from build123d import *

# Parameters (mm, degrees)
SKETCH1_R               = 387.5
BOSS_EXTRUDE1_DEPTH     = 62
SKETCH3_R               = 17.4625
CUT_EXTRUDE1_DEPTH      = 552.503853114
SKETCH2_R               = 292.1
BOSS_EXTRUDE2_DEPTH     = 1.5
CIRPATTERN1_COUNT       = 24
CUT_EXTRUDE4_DEPTH      = 552.67449642
CUT_EXTRUDE4_DEPTH_BACK = 552.67449642
SKETCH8_R               = 292.1


with BuildPart() as part:
    # Sketch1 → Boss-Extrude1 (new body)
    with BuildSketch(Plane.XY):
        Circle(SKETCH1_R)
    extrude(amount=BOSS_EXTRUDE1_DEPTH)

    # Sketch3 → Cut-Extrude1 (cut, symmetric)
    with BuildSketch(Plane.XY.offset(62)):
        with Locations((0, 342.9)):
            Circle(SKETCH3_R)
    cut_extrude1 = extrude(amount=CUT_EXTRUDE1_DEPTH, both=True, mode=Mode.SUBTRACT)

    # Sketch2 → Boss-Extrude2 (add)
    with BuildSketch(Plane.XY.offset(62)):
        Circle(SKETCH2_R)
    extrude(amount=BOSS_EXTRUDE2_DEPTH)

    # CirPattern1: Cut-Extrude1 ×24 about axis
    cirpattern1_axis = Axis((0, 0, 0), (0, 0, 1))
    for i in range(1, CIRPATTERN1_COUNT):
        add(cut_extrude1.rotate(cirpattern1_axis, i * 360 / CIRPATTERN1_COUNT), mode=Mode.SUBTRACT)

    # Sketch8 → Cut-Extrude4 (cut, two sides: drawn at the far end of the back side and taken through both)
    with BuildSketch(Plane.XY.offset(63.5).offset(-CUT_EXTRUDE4_DEPTH_BACK)):
        Circle(SKETCH8_R)
    extrude(amount=CUT_EXTRUDE4_DEPTH + CUT_EXTRUDE4_DEPTH_BACK, mode=Mode.SUBTRACT)


solid = part.part
CAD build for the part. Positions are in the model's coordinates, mm. Coordinates: 2 decimals unless noted, no trailing zeros. Order: outer loops, then holes, each group sorted by start corner. A loop starts at its lowest first (then second) coordinate and runs counter-clockwise, first axis right, second up.
Item 1: Pin check, flat tips, straight feed: pin 1 Ø21 at (x, y) = (331.22, 88.75) entering from +Z; pin 2 Ø3 at (x, z) = (82.5, 55.5) entering from -Y; pin 3 Ø5 at (y, z) = (301, 14) entering from +X; pin 4 Ø1 at (x, z) = (247, 27) entering from +Y. Stop position of each tip, or through.
Check sheet entries:
pin 1: passes through
pin 2: stops at y = -378.94
pin 3: stops at x = 247.09
pin 4: stops at y = 298.99
Item 2: Band-saw the part on C-C on z = 41. Give the number of separate pieces and of enclosed holes in the cut face, plus the area to 3 significant figures.
Check sheet entries:
separate pieces: 1
enclosed holes: 25
area: 181,000 mm2
Item 3: Band-saw the part on A-A on x = 0. List the corners of the cut face in (y, z), plus the area to 3 significant figures.
Check sheet entries:
outline: (-387.5, 0) - (-360.36, 0) - (-360.36, 62) - (-387.5, 62) - close; (-325.44, 0) - (-292.1, 0) - (-292.1, 62) - (-325.44, 62) - close; (292.1, 0) - (325.44, 0) - (325.44, 62) - (292.1, 62) - close; (360.36, 0) - (387.5, 0) - (387.5, 62) - (360.36, 62) - close
area: 7,500 mm2
Item 4: Band-saw the part on B-B on y = -171.45. List the corners of the cut face in (x, z), plus the area to 3 significant figures.
Check sheet entries:
outline: (-347.51, 0) - (-314.42, 0) - (-314.42, 62) - (-347.51, 62) - close; (-279.5, 0) - (-236.49, 0) - (-236.49, 62) - (-279.5, 62) - close; (236.49, 0) - (279.5, 0) - (279.5, 62) - (236.49, 62) - close; (314.42, 0) - (347.51, 0) - (347.51, 62) - (314.42, 62) - close
area: 9,440 mm2
Item 5: Two-plate mould, pull along Y, no slides. Class faces 1 (the face through (2.273, -360.214, 31.434)), 2 (the face through (56, 289, 0)): +Y half, -Y half, draft (parallel to the pull), parting line (faces both ways), or undercut.
Check sheet entries:
face 1: undercut
face 2: draft
Item 6: Drill centre lines: L1, parallel to Y at x = 0, z = 40.5; L2, parallel to Y at x = 251, z = 39.5; L3, parallel to Y at x = -293.5, z = 48. Where is each one in solid material? Low to high.
Check sheet entries:
L1: y = -387.5 to -360.36, -325.44 to -292.1, 292.1 to 325.44, 360.36 to 387.5
L2: y = -295.22 to -257.7, -227.23 to -149.4, 149.4 to 227.23, 257.7 to 295.22
L3: y = -253.01 to -188.57, -154.33 to 154.33, 188.57 to 253.01
